Here's how the part is built. I have some questions about the finished solid (model axes, mm). Round coordinates to 2 decimals unless told otherwise and drop trailing zeros. Write each loop counter-clockwise with the first axis right and the second up, starting at its lowest first coordinate (ties: lowest second). Pieces come first, ordered by that corner, then holes. Notation, with made-up numbers: (31, 20.5) - (86, 20.5) arc R18 cw to (86, 41.5) - close; hole circle Ø11 at (30, 33). An arc over 180 degrees is marked (long way). One line per item, written item: value. Start each with the question number.
Item 1: Imagine slicing it at C-C, the plane z = -0.2. Please give me the cut outline in (x, y), then the cut area to 3 significant figures.
Item 2: For P1, Ø5.5, axis at x = -19.05, y = 19.05, coming from the +Z side (3 decimals), with a flat end and sliding along its axis, tell me the tip position at first contact or that it passes through.
Item 3: Thinking about a two-plate mould opening in X: for faces 1 (the face through (0, 25.4, 0)), 2 (the face through (-17.958, -17.337, -0.009)), 3 (the face through (25.4, 0, 0)), which applies, released by +X, released by -X, zero draft, split by the parting line, or undercut?
Item 4: Imagine slicing it at A-A, the plane x = 0. Please give me the cut outline in (y, z) (3 decimals).
Item 5: If I drill on line 1 (Y direction, x = -19.05, z = 0.1); line 2 (Y direction, x = 19.5, z = -0.35); line 3 (X direction, y = -17.5, z = -0.6), over which ranges is the centre line in solid material (lowest first)?
Item 6: Imagine slicing it at B-B, the plane y = -19.05. Please give me the cut outline in (x, z) (3 decimals).
```python
from build123d import *

# Parameters (mm, degrees)
SKETCH1_W           = 50.8
SKETCH1_H           = 50.8
SKETCH1_R           = 14.351
SKETCH1_R_2         = 2.032
BOSS_EXTRUDE1_DEPTH = 0.635


with BuildPart() as part:
    # Sketch1 → Boss-Extrude1 (new, symmetric)
    with BuildSketch(Plane.XY):
        Rectangle(SKETCH1_W, SKETCH1_H)
        Circle(SKETCH1_R, mode=Mode.SUBTRACT)
        with Locations((19.05, 19.05)):
            Circle(SKETCH1_R_2, mode=Mode.SUBTRACT)
        with Locations(Location((-19.05, 19.05, 0), (0, 0, 180))):
            Circle(SKETCH1_R_2, mode=Mode.SUBTRACT)
        with Locations(Location((19.05, -19.05, 0), (0, 0, 180))):
            Circle(SKETCH1_R_2, mode=Mode.SUBTRACT)
        with Locations((-19.05, -19.05)):
            Circle(SKETCH1_R_2, mode=Mode.SUBTRACT)
    extrude(amount=BOSS_EXTRUDE1_DEPTH, both=True)


solid = part.part
```
Values follow:
1. outline: (-25.4, -25.4) - (25.4, -25.4) - (25.4, 25.4) - (-25.4, 25.4) - close; hole circle Ø4.06 at (-19.05, -19.05); hole circle Ø4.06 at (-19.05, 19.05); hole circle Ø28.7 at (0, 0); hole circle Ø4.06 at (19.05, -19.05); hole circle Ø4.06 at (19.05, 19.05)
1. area: 1,880 mm^2
2. P1: stops at z = 0.635
3. face 1: zero draft
3. face 2: undercut
3. face 3: released by +X
4. outline: (-25.4, -0.635) - (-14.351, -0.635) - (-14.351, 0.635) - (-25.4, 0.635) - close; (14.351, -0.635) - (25.4, -0.635) - (25.4, 0.635) - (14.351, 0.635) - close
5. line 1: y = -25.4 to -21.08, -17.02 to 17.02, 21.08 to 25.4
5. line 2: y = -25.4 to -21.03, -17.07 to 17.07, 21.03 to 25.4
5. line 3: x = -25.4 to -20.36, -17.74 to 17.74, 20.36 to 25.4
6. outline: (-25.4, -0.635) - (-21.082, -0.635) - (-21.082, 0.635) - (-25.4, 0.635) - close; (-17.018, -0.635) - (17.018, -0.635) - (17.018, 0.635) - (-17.018, 0.635) - close; (21.082, -0.635) - (25.4, -0.635) - (25.4, 0.635) - (21.082, 0.635) - close
